from build123d import *

# Parameters (mm, degrees)
BOSS_EXTRUDE1_DEPTH = 8


with BuildPart() as part:
    # Sketch2 → Boss-Extrude1 (new body)
    with BuildSketch(Plane(origin=(0, 0, 0), x_dir=(1, 0, 0), z_dir=(0, 1, 0))):
        with BuildLine():
            ThreePointArc((-7.544444444, -2.948110925), (0, -8.1), (7.544444444, -2.948110925))
            ThreePointArc((7.544444444, -2.948110925), (11.1, 0), (7.544444444, 2.948110925))
            ThreePointArc((7.544444444, 2.948110925), (0, 8.1), (-7.544444444, 2.948110925))
            ThreePointArc((-7.544444444, 2.948110925), (-11.1, 0), (-7.544444444, -2.948110925))
        make_face()
    extrude(amount=-BOSS_EXTRUDE1_DEPTH)

    # Sketch3 → Revolve1 (revolve)
    with BuildSketch(Plane.XZ.offset(8)):
        with BuildLine():
            Line((0, 7), (0, -7))
            ThreePointArc((0, -7), (-7, 0), (0, 7))
        make_face()
    revolve(axis=Axis((0, -8, 7), (0, 0, -1)))


solid = part.part
Check sheet for the modelled part. Datum: model origin and axes. Units: mm. A direction names the side the tool comes from. Round coordinates to 2 decimals unless told otherwise and drop trailing zeros. Loops run counter-clockwise (first coordinate to the right, second up) from the corner with the lowest first, then second, coordinate; pieces in that order, holes last. Notation, with made-up numbers: (81.5, 27) - (109.5, 27) arc R14 cw to (109.5, 39) - close; hole circle Ø5 at (83.5, 19). An arc over 180 degrees is marked (long way). Answer as CSV lines item,"result". Start each with the question number.
Item 1: Set-up check for faces 1 (the flat face through (-3, -8, 7)), 2 (the cylindrical face through (-0.1, -3.9, 8.1)): record each of +Z, -Z, +X, -X, +Y, -Y from which the full face is reachable in a straight line by a thin tool's end or side.
Item 2: Section check A-A (z = 0). Record the boundary of the cut face in (x, y).
Item 3: Section check B-B (x = -5.5). Record the boundary of the cut face in (y, z), and give its area (3 significant figures).
Item 4: Depth check by flat-ended pin: P1, Ø1, axis at x = 3.5, z = -1.5, coming from the -Y side; P2, Ø5, axis at x = -5.5, z = 2, coming from the -Y side; P3, Ø5, axis at y = -11, z = 3, coming from the -X side. Enter the tip coordinate at first touch or a pass-through.
Item 5: Scan lines: line 1 (Y direction, x = 7, z = 2.5); line 2 (Z direction, x = 8, y = -5.25); line 3 (X direction, y = -2.25, z = 4.25). Record each from-to range of solid material in increasing order. Write a range as [from, to].
Item 6: Section check C-C (y = -2). Record the boundary of the cut face in (x, z), and give its area (3 significant figures).
Item 7: Section check D-D (x = 8.1). Record the boundary of the cut face in (y, z), and give its area (3 significant figures).
Report:
1,face 1,"-Y"
1,face 2,"+Z, +Y, -Y"
2,outline,"(-11.1, -8) - (-7, -8) arc R7 ccw to (7, -8) - (11.1, -8) - (11.1, 0) - (-11.1, 0) - close"
3,outline,"(-8, -5.95) - (0, -5.95) - (0, 5.95) - (-8, 5.95) - (-8, 4.33) arc R4.33 ccw to (-8, -4.33) - close"
3,area,"125 mm2"
4,P1,"stops at y = -14.17"
4,P2,"stops at y = -14.15"
4,P3,"stops at x = -6.78"
5,line 1,"y = [-8, 0]"
5,line 2,"z = [-3, 3]"
5,line 3,"x = [-6.9, 6.9]"
6,outline,"(-7.54, -2.95) arc R8.1 ccw to (7.54, -2.95) arc R3 ccw (long way) to (7.54, 2.95) arc R8.1 ccw to (-7.54, 2.95) arc R3 ccw (long way) to start"
6,area,"237 mm2"
7,outline,"(-8, -3) - (0, -3) - (0, 3) - (-8, 3) - close"
7,area,"48.0 mm2"
